Part model, mm, in its own coordinate system. Face numbers are marked on the shaded views. Give positions to 0.01 mm unless a question says otherwise; leave off trailing zeros. Write each loop counter-clockwise with the first axis right and the second up, starting at its lowest first coordinate (ties: lowest second). Pieces come first, ordered by that corner, then holes. Notation, with made-up numbers: M 75.5,-30.5 L 103.5,-30.5 A10 cw 103.5,-14.5 Z; hole C 27,-29.5 d7. An arc over 180 degrees is marked long. Answer as CSV lines item,"result". Start each with the question number.
Item 1: Pin check, flat tips, straight feed: pin 1 (2.5 mm diameter, centred on x = 28.5, y = 2, fed in from +Z); pin 2 (1 mm diameter, centred on x = 97.5, z = 11, fed in from +Y); pin 3 (24.5 mm diameter, centred on x = -170.5, z = 32, fed in from +Y); pin 4 (4.5 mm diameter, centred on x = 177.8, z = 63.5, fed in from -Y). Stop position of each tip, or through.
Item 2: Band-saw the part on C-C, the plane y = 38.5. List the corners of the cut face in (x, z).
Item 3: Band-saw the part on B-B, the plane x = -70.5. List the corners of the cut face in (y, z) (1 decimal).
Item 4: Two-plate mould, pull along Y, no slides. Class the marked faces 1, 2 and 3: +Y half, -Y half, draft (parallel to the pull), parting line (faces both ways), or undercut.
Item 5: Wall check: L1, parallel to X at y = 1, z = 50; L2, parallel to Y at x = 82.5, z = 12; L3, parallel to Z at x = 126.5, y = 48.5. Give the ranges that are in metal, low to high. Write a range as from..to.
Item 6: Band-saw the part on A-A, the plane z = 28. List the corners of the cut face in (x, y), then the cut area to 3 significant figures.
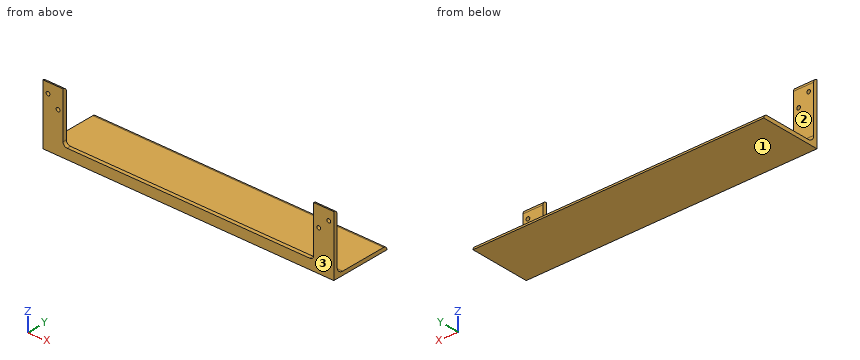
from build123d import *

# Parameters (mm, degrees)
F1_DEPTH = 184.15
F2_W     = 317.5
F2_H     = 68.2625
F2_H_2   = 58.7375
F3_DEPTH = 4.7635
F4_R     = 5.08
F5_R     = 2.38125
F6_DEPTH = 76.201


with BuildPart() as f1:
    # F0 (on Right) → F1 (new body, symmetric)
    with BuildSketch(Plane.YZ):
        with BuildLine():
            ThreePointArc((4.7625, 71.4375), (3.3675960454, 74.8050960454), (0, 76.2))
            Line((0, 76.2), (0, 0))
            Line((0, 0), (76.2, 0))
            ThreePointArc((76.2, 0), (74.8050960454, 3.3675960454), (71.4375, 4.7625))
            Line((71.4375, 4.7625), (12.7, 4.7625))
            ThreePointArc((12.7, 4.7625), (7.0873399243, 7.0873399243), (4.7625, 12.7))
            Line((4.7625, 12.7), (4.7625, 71.4375))
        make_face()
    extrude(amount=F1_DEPTH, both=True)

    # F2 (on face) → F3 (cut, through all)
    with BuildSketch(Plane(origin=(0, 4.7625, 0), x_dir=(-1, 0, 0), z_dir=(0, 1, 0))):
        with Locations((0, 105.56875)):
            Rectangle(F2_W, F2_H)
        with Locations((0, 42.06875)):
            Rectangle(F2_W, F2_H_2)
    extrude(amount=-F3_DEPTH, mode=Mode.SUBTRACT)

    # F4
    f4_edges = [f1.edges().sort_by_distance(p)[0] for p in [
        (158.75, 2.38125, 12.7),
        (-158.75, 2.38125, 12.7),
    ]]
    fillet(f4_edges, radius=F4_R)

    # F5 (on face) → F6 (cut, through all)
    with BuildSketch(Plane.XZ):
        with Locations((-165.1, 50.8)):
            Circle(F5_R)
        with Locations((-177.8, 63.5)):
            Circle(F5_R)
        with Locations((177.8, 63.5)):
            Circle(F5_R)
        with Locations((165.1, 50.8)):
            Circle(F5_R)
    extrude(amount=-F6_DEPTH, mode=Mode.SUBTRACT)


solid = f1.part
Output:
1,pin 1,"z = 12.7"
1,pin 2,"y = 5.07"
1,pin 3,"y = 4.76"
1,pin 4,"through"
2,outline,"M -184.15,0 L 184.15,0 L 184.15,4.76 L -184.15,4.76 Z"
3,outline,"M 0,0 L 76.2,0 A4.8 ccw 71.4,4.8 L 12.7,4.8 A7.9 cw 4.8,12.7 L 0,12.7 Z"
4,face 1,"draft"
4,face 2,"+Y half"
4,face 3,"-Y half"
5,L1,"-184.15..-167.34, -162.86..-158.75, 158.75..162.86, 167.34..184.15"
5,L2,"0..4.79"
5,L3,"0..4.76"
6,outline,"M -184.15,0 L -158.75,0 L -158.75,4.76 L -184.15,4.76 Z; M 158.75,0 L 184.15,0 L 184.15,4.76 L 158.75,4.76 Z"
6,area,"242 mm²"
